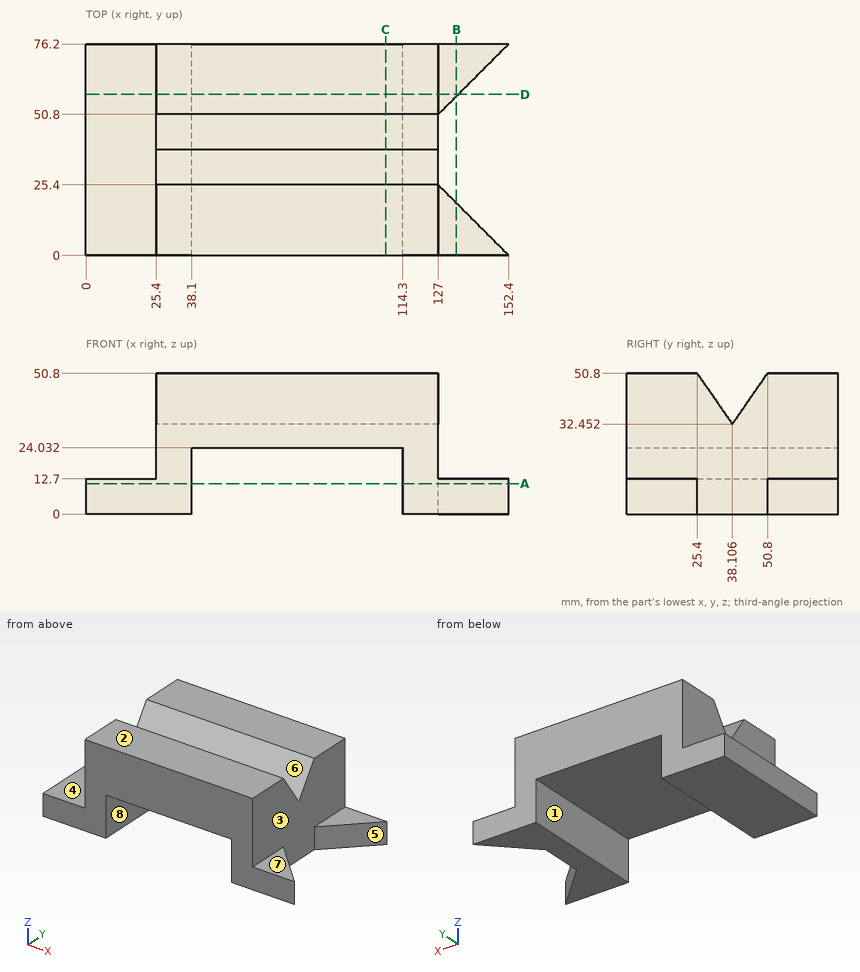
Here's the drawing with two shaded views (mm, measured from the low corner). I have some questions. A direction names the side the tool comes from. Coordinates: 2 decimals unless noted, no trailing zeros. Loops run counter-clockwise (first coordinate to the right, second up) from the corner with the lowest first, then second, coordinate; pieces in that order, holes last. Notation, with made-up numbers: (85.25, 61) -> (136.25, 61) arc R16 ccw to (136.25, 67) -> close; hole circle Ø10 at (67.25, 53.5). An arc over 180 degrees is marked (long way). Answer as a JSON object with one key per item and string values.
1) For the marked faces 4, 5, 6, 7 and 8, which set-ups out of +Z, -Z, +X, -X, +Y, -Y let a thin tool reach every point of the face, with its end or its side?
Results:
{"face 4": "+Z, -X, +Y, -Y", "face 5": "+Z, -Z, +X", "face 6": "+Z, +X, -X", "face 7": "+Z, +X, +Y, -Y", "face 8": "-Z, +Y, -Y"}
2) If I drill on line 1 (X direction, y = 36.5, z = 16); line 2 (X direction, y = 26, z = 27); line 3 (Z direction, x = 89.5, y = 18), over which ranges is the centre line in solid material (lowest first)?
Results:
{"line 1": "x = 25.4 to 38.1, 114.3 to 127", "line 2": "x = 25.4 to 127", "line 3": "z = 24.03 to 50.8"}
3) Imagine slicing it at B-B (x = 133.5). Please give me the cut outline in (y, z).
Results:
{"outline": "(0, 0) -> (18.9, 0) -> (18.9, 12.7) -> (0, 12.7) -> close; (57.3, 0) -> (76.2, 0) -> (76.2, 12.7) -> (57.3, 12.7) -> close"}
4) For P1, Ø1.5, axis at y = 19, z = 6, coming from the +X side; P2, Ø6, axis at y = 39.5, z = 15.5, coming from the +X side; P3, Ø12.5, axis at x = 14, y = 46.5, coming from the +Z side; P4, Ø5, axis at x = 27, z = 7.5, coming from the -Y side, each with a flat end and sliding along its axis, tell me the tip position at first contact or that it passes through.
Results:
{"P1": "stops at x = 134.15", "P2": "stops at x = 127", "P3": "stops at z = 12.7", "P4": "stops at y = 0"}
5) Imagine slicing it at D-D (y = 58). Please give me the cut outline in (x, z), then the cut area to 3 significant figures.
Results:
{"outline": "(0, 0) -> (38.1, 0) -> (38.1, 24.03) -> (114.3, 24.03) -> (114.3, 0) -> (134.2, 0) -> (134.2, 12.7) -> (127, 12.7) -> (127, 50.8) -> (25.4, 50.8) -> (25.4, 12.7) -> (0, 12.7) -> close", "area": "3,740 mm^2"}
6) Thinking about a two-plate mould opening in X: for the marked faces 1, 2 and 3, which applies, pulls with the +X half, pulls with the -X half, needs draft (parallel to the pull), parting line crosses it, or undercut?
Results:
{"face 1": "undercut", "face 2": "needs draft", "face 3": "pulls with the +X half"}
7) Imagine slicing it at A-A (z = 11). Please give me the cut outline in (x, y).
Results:
{"outline": "(0, 0) -> (38.1, 0) -> (38.1, 76.2) -> (0, 76.2) -> close; (114.3, 0) -> (152.4, 0) -> (127, 25.4) -> (127, 50.8) -> (152.4, 76.2) -> (114.3, 76.2) -> close"}
8) Imagine slicing it at C-C (x = 108). Please give me the cut outline in (y, z).
Results:
{"outline": "(0, 24.03) -> (76.2, 24.03) -> (76.2, 50.8) -> (50.8, 50.8) -> (38.11, 32.45) -> (25.4, 50.8) -> (0, 50.8) -> close"}
